from build123d import *

# Parameters (mm, degrees)
EXTRUDE_1_DEPTH        = 280
SKETCH_2_R             = 5.5
CUT_EXTRUDE_1_DEPTH    = 9
SKETCH_3_R             = 3.5
CUT_EXTRUDE_2_DEPTH    = 281.699127181
PATTERN_LINEAR_1_COUNT = 4
PATTERN_LINEAR_1_PITCH = 80


with BuildPart() as part:
    # 草图1 → 凸台-拉伸1 (new body)
    with BuildSketch(Plane(origin=(0, 0, 0), x_dir=(1, 0, 0), z_dir=(0, 1, 0))):
        with BuildLine():
            Line((11.758193654, -0.458193653), (11.300000001, 0))
            Line((11.300000001, 0), (-11.299999999, 0))
            Line((-11.299999999, 0), (-11.758193652, -0.458193653))
            ThreePointArc((-11.758193652, -0.458193653), (-11.768448168, -0.468969729), (-11.778155913, -0.480240869))
            ThreePointArc((-11.778155913, -0.480240869), (-12.478076595, -1.902541611), (-13.892618036, -2.618014092))
            ThreePointArc((-13.892618036, -2.618014092), (-13.971832127, -2.721095863), (-13.999999999, -2.848010379))
            Line((-13.999999999, -2.848010379), (-13.999999999, -5.15198962))
            ThreePointArc((-13.999999999, -5.15198962), (-13.971832127, -5.278904137), (-13.892618036, -5.381985907))
            ThreePointArc((-13.892618036, -5.381985907), (-12.478076595, -6.097458389), (-11.778155913, -7.519759131))
            ThreePointArc((-11.778155913, -7.519759131), (-11.768448168, -7.531030271), (-11.758193652, -7.541806347))
            Line((-11.758193652, -7.541806347), (-10.939339827, -8.360660172))
            ThreePointArc((-10.939339827, -8.360660172), (-10.614191318, -8.847269563), (-10.5, -9.421264856))
            Line((-10.5, -9.421264856), (-10.5, -11.878679656))
            ThreePointArc((-10.5, -11.878679656), (-10.614180701, -12.452704805), (-10.939339828, -12.939339828))
            Line((-10.939339828, -12.939339828), (-13.560660172, -15.560660172))
            ThreePointArc((-13.560660172, -15.560660172), (-13.88581399, -16.047282379), (-14, -16.6212926))
            Line((-14, -16.6212926), (-14, -21.5))
            Line((-14, -21.5), (-12.5, -23))
            Line((-12.5, -23), (-5, -23))
            Line((-5, -23), (-4.5, -22.5))
            Line((-4.5, -22.5), (4.5, -22.5))
            Line((4.5, -22.5), (5, -23))
            Line((5, -23), (12.5, -23))
            Line((12.5, -23), (14, -21.5))
            Line((14, -21.5), (14, -16.621320344))
            ThreePointArc((14, -16.621320344), (13.885819299, -16.047295195), (13.560660172, -15.560660172))
            Line((13.560660172, -15.560660172), (10.939339828, -12.939339828))
            ThreePointArc((10.939339828, -12.939339828), (10.61418601, -12.452717621), (10.5, -11.8787074))
            Line((10.5, -11.8787074), (10.5, -9.421320344))
            ThreePointArc((10.5, -9.421320344), (10.614180701, -8.847295195), (10.939339828, -8.360660172))
            Line((10.939339828, -8.360660172), (11.758193653, -7.541806347))
            ThreePointArc((11.758193653, -7.541806347), (11.768448169, -7.531030271), (11.778155914, -7.519759131))
            ThreePointArc((11.778155914, -7.519759131), (12.478076596, -6.097458389), (13.892618037, -5.381985908))
            ThreePointArc((13.892618037, -5.381985908), (13.971832128, -5.278904137), (14, -5.15198962))
            Line((14, -5.15198962), (14, -2.848010379))
            ThreePointArc((14, -2.848010379), (13.971832128, -2.721095863), (13.892618037, -2.618014092))
            ThreePointArc((13.892618037, -2.618014092), (12.478076596, -1.902541611), (11.778155915, -0.480240869))
            ThreePointArc((11.778155915, -0.480240869), (11.76844817, -0.468969728), (11.758193654, -0.458193653))
        make_face()
    extrude(amount=EXTRUDE_1_DEPTH)

    # 草图2 → 切除-拉伸1 (cut)
    with BuildSketch(Plane(origin=(0, 0, 0), x_dir=(-1, 0, 0), z_dir=(0, 0, -1))):
        with Locations((0, 50)):
            Circle(SKETCH_2_R)
    cut_extrude_1 = extrude(amount=-CUT_EXTRUDE_1_DEPTH, mode=Mode.SUBTRACT)

    # 草图3 → 切除-拉伸2 (cut, through all)
    with BuildSketch(Plane(origin=(0, 0, 9), x_dir=(-1, 0, 0), z_dir=(0, 0, -1))):
        with Locations((0, 50)):
            Circle(SKETCH_3_R)
    cut_extrude_2 = extrude(amount=-CUT_EXTRUDE_2_DEPTH, mode=Mode.SUBTRACT)

    # 阵列(线性)1: 切除-拉伸1, 切除-拉伸2 ×4
    with Locations(*[(0, i * PATTERN_LINEAR_1_PITCH, 0) for i in range(1, PATTERN_LINEAR_1_COUNT)]):
        add(cut_extrude_1, mode=Mode.SUBTRACT)
        add(cut_extrude_2, mode=Mode.SUBTRACT)


solid = part.part
The listing builds one solid part. Answer for the finished solid, in the listing's coordinates (mm). A direction names the side the tool comes from. Give positions to 0.01 mm unless a question says otherwise; leave off trailing zeros. Write each loop counter-clockwise with the first axis right and the second up, starting at its lowest first coordinate (ties: lowest second). Pieces come first, ordered by that corner, then holes. Notation, with made-up numbers: (1, 57) - (37, 57) arc R23 cw to (37, 85) - close; hole circle Ø7 at (-23.75, 87). An arc over 180 degrees is marked (long way). Use a Markdown table: item, result.
1. Section A-A on x = 0 is taken. Write down the section's boundary in (y, z), plus the area to 3 significant figures.
Values follow:
| item | result |
|---|---|
| outline | (0, 0) - (44.5, 0) - (44.5, 9) - (46.5, 9) - (46.5, 22.5) - (0, 22.5) - close; (53.5, 9) - (55.5, 9) - (55.5, 0) - (124.5, 0) - (124.5, 9) - (126.5, 9) - (126.5, 22.5) - (53.5, 22.5) - close; (133.5, 9) - (135.5, 9) - (135.5, 0) - (204.5, 0) - (204.5, 9) - (206.5, 9) - (206.5, 22.5) - (133.5, 22.5) - close; (213.5, 9) - (215.5, 9) - (215.5, 0) - (280, 0) - (280, 22.5) - (213.5, 22.5) - close |
| area | 5,720 mm² |
2. A tool of negligible diameter and unlimited length cuts with its end or side. For faces 1 (the cylindrical face through (1.19, 204.63, 4.44)), 2 (the flat face through (-14, 138, 19)), 3 (the flat face through (0, 138, 22.5)), from which of +Z, -Z, +X, -X, +Y, -Y can it reach the whole face along a straight path? Write none if from no direction.
Values follow:
| item | result |
|---|---|
| face 1 | -Z |
| face 2 | +Z, -Z, -X, +Y, -Y |
| face 3 | +Z, +Y, -Y |
3. Each of these flat-tipped pins is pushed along its axis until it touches: P1, Ø1.2, axis at y = 93.5, z = 10.5, coming from the -X side; P2, Ø9, axis at x = 0, y = 50, coming from the -Z side; P3, Ø8, axis at x = 0, y = 130, coming from the +Z side; P4, Ø5.5, axis at x = 0, y = 50, coming from the -Z side. Where does it stop, or does it pass through?
Values follow:
| item | result |
|---|---|
| P1 | stops at x = -10.5 |
| P2 | stops at z = 9 |
| P3 | stops at z = 22.5 |
| P4 | passes through |
4. For a pull along X with two mould halves and no side action, classify faces 4 (the flat face through (14, 138, 19)), 5 (the flat face through (-9, 138, 23)), 6 (the flat face through (-4, 210, 9)) as released by +X, released by -X, zero draft, split by the parting line, or undercut.
Values follow:
| item | result |
|---|---|
| face 4 | released by +X |
| face 5 | zero draft |
| face 6 | undercut |
5. Find the intervals of material crossed by probe 1 along Y at (x, z) = (0, 13.75); probe 2 along Y at (x, z) = (0, 6); probe 3 along X at (y, z) = (210, 19.5), in increasing order. Write a range as from..to.
Values follow:
| item | result |
|---|---|
| probe 1 | y = 0..46.5, 53.5..126.5, 133.5..206.5, 213.5..280 |
| probe 2 | y = 0..44.5, 55.5..124.5, 135.5..204.5, 215.5..280 |
| probe 3 | x = -14..-3.5, 3.5..14 |
